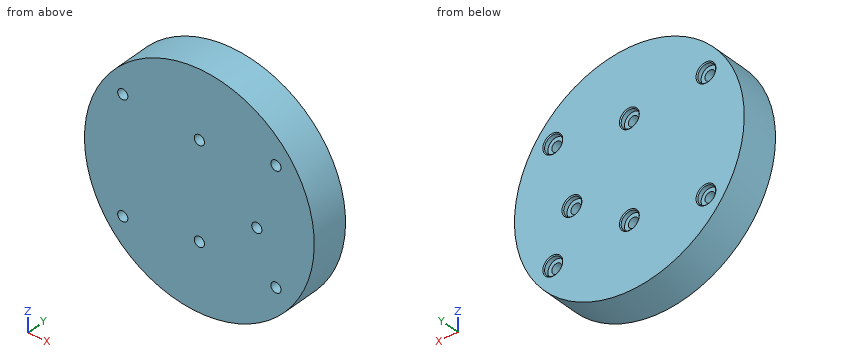
from build123d import *

# Parameters (mm, degrees)
SKETCH1_R                                     = 76.2
BOSS_EXTRUDE1_DEPTH                           = 25.4
CBORE_FOR_1_4_BUTTON_HEAD_CAP_SCREW1_AT_COUNT = 2
CBORE_FOR_1_4_BUTTON_HEAD_CAP_SCREW1_AT_PITCH = 45.790501198
CBORE_FOR_1_4_BUTTON_HEAD_CAP_SCREW1_2_COUNT  = 2
CBORE_FOR_1_4_BUTTON_HEAD_CAP_SCREW1_2_PITCH  = 63.5
CBORE_FOR_1_4_BUTTON_HEAD_CAP_SCREW1_3_COUNT  = 2
CBORE_FOR_1_4_BUTTON_HEAD_CAP_SCREW1_3_PITCH  = 86.36933773
CBORE_FOR_1_4_BUTTON_HEAD_CAP_SCREW1_4_COUNT  = 2
CBORE_FOR_1_4_BUTTON_HEAD_CAP_SCREW1_4_PITCH  = 51.195336702
CBORE_FOR_1_4_BUTTON_HEAD_CAP_SCREW1_5_COUNT  = 2
CBORE_FOR_1_4_BUTTON_HEAD_CAP_SCREW1_5_PITCH  = 51.195336702
CBORE_FOR_1_4_BUTTON_HEAD_CAP_SCREW1_6_COUNT  = 2
CBORE_FOR_1_4_BUTTON_HEAD_CAP_SCREW1_6_PITCH  = 86.36933773


with BuildPart() as part:
    # Sketch1 → Boss-Extrude1 (new body)
    with BuildSketch(Plane(origin=(0, 0, 0), x_dir=(1, 0, 0), z_dir=(0, 1, 0))):
        with Locations(Location((0, 0, 0), (0, 0, 270))):
            Circle(SKETCH1_R)
    extrude(amount=-BOSS_EXTRUDE1_DEPTH)

    # Sketch8 → CBORE for 1/4 Button Head Cap Screw1 (revolve, cut)
    with BuildSketch(Plane(origin=(0, 0, -31.75), x_dir=(0, 0, 1), z_dir=(1, 0, 0))):
        Polygon((0, 0), (0, 25.4), (3.3782, 25.4), (3.3782, 3.3528), (5.95376, 3.3528), (5.95376, 0.635), (6.58876, 0), align=None)
    cbore_for_1_4_button_head_cap_screw1 = revolve(axis=Axis((0, 6.35, -31.75), (0, -1, 0)), mode=Mode.SUBTRACT)

    # CBORE for 1/4 Button Head Cap Screw1 at: CBORE for 1/4 Button Head Cap Screw1 ×2
    with Locations(*[Vector(0.8320502943378437, 0, 0.5547001962252293) * (i * CBORE_FOR_1_4_BUTTON_HEAD_CAP_SCREW1_AT_PITCH) for i in range(1, CBORE_FOR_1_4_BUTTON_HEAD_CAP_SCREW1_AT_COUNT)]):
        add(cbore_for_1_4_button_head_cap_screw1, mode=Mode.SUBTRACT)

    # CBORE for 1_4 Button Head Cap Screw1 2: CBORE for 1/4 Button Head Cap Screw1 ×2
    with Locations(*[(0, 0, i * CBORE_FOR_1_4_BUTTON_HEAD_CAP_SCREW1_2_PITCH) for i in range(1, CBORE_FOR_1_4_BUTTON_HEAD_CAP_SCREW1_2_COUNT)]):
        add(cbore_for_1_4_button_head_cap_screw1, mode=Mode.SUBTRACT)

    # CBORE for 1_4 Button Head Cap Screw1 3: CBORE for 1/4 Button Head Cap Screw1 ×2
    with Locations(*[Vector(0.5881716976750462, 0, 0.8087360843031886) * (i * CBORE_FOR_1_4_BUTTON_HEAD_CAP_SCREW1_3_PITCH) for i in range(1, CBORE_FOR_1_4_BUTTON_HEAD_CAP_SCREW1_3_COUNT)]):
        add(cbore_for_1_4_button_head_cap_screw1, mode=Mode.SUBTRACT)

    # CBORE for 1_4 Button Head Cap Screw1 4: CBORE for 1/4 Button Head Cap Screw1 ×2
    with Locations(*[Vector(0.9922778767136676, 0, -0.12403473458920865) * (i * CBORE_FOR_1_4_BUTTON_HEAD_CAP_SCREW1_4_PITCH) for i in range(1, CBORE_FOR_1_4_BUTTON_HEAD_CAP_SCREW1_4_COUNT)]):
        add(cbore_for_1_4_button_head_cap_screw1, mode=Mode.SUBTRACT)

    # CBORE for 1_4 Button Head Cap Screw1 5: CBORE for 1/4 Button Head Cap Screw1 ×2
    with Locations(*[Vector(-0.9922778767136676, 0, -0.12403473458920862) * (i * CBORE_FOR_1_4_BUTTON_HEAD_CAP_SCREW1_5_PITCH) for i in range(1, CBORE_FOR_1_4_BUTTON_HEAD_CAP_SCREW1_5_COUNT)]):
        add(cbore_for_1_4_button_head_cap_screw1, mode=Mode.SUBTRACT)

    # CBORE for 1_4 Button Head Cap Screw1 6: CBORE for 1/4 Button Head Cap Screw1 ×2
    with Locations(*[Vector(-0.5881716976750463, 0, 0.8087360843031884) * (i * CBORE_FOR_1_4_BUTTON_HEAD_CAP_SCREW1_6_PITCH) for i in range(1, CBORE_FOR_1_4_BUTTON_HEAD_CAP_SCREW1_6_COUNT)]):
        add(cbore_for_1_4_button_head_cap_screw1, mode=Mode.SUBTRACT)


solid = part.part
The listing builds one solid part. Answer for the finished solid, in the listing's coordinates (mm). Coordinates: 2 decimals unless noted, no trailing zeros. Write each loop counter-clockwise with the first axis right and the second up, starting at its lowest first coordinate (ties: lowest second). Pieces come first, ordered by that corner, then holes. Notation, with made-up numbers: (-38, 6) -> (-2, 6) arc R37 cw to (-2, 45) -> close; hole circle Ø2 at (14.25, 84). An arc over 180 degrees is marked (long way). One line per question, with ' | ' between items.
1. Straight lines are drawn through the part: line 1 (Z direction, x = -53.5, y = -8); line 2 (Z direction, x = 52.5, y = -18); line 3 (X direction, y = -2.3, z = -6.35). For each, find the intervals that lie inside material, in ascending order.
Verdict:
line 1: z = -54.26 to -40.13, -36.07 to 36.07, 40.13 to 54.26 | line 2: z = -55.23 to -41.02, -35.18 to 35.18, 41.02 to 55.23 | line 3: x = -75.93 to 32.15, 44.05 to 75.93
2. Section A-A (x = 0) is taken. Determine the outline of the cut face in (y, z) (3 decimals), and give its area (3 significant figures).
Verdict:
outline: (-25.4, -76.2) -> (0, -76.2) -> (0, -38.339) -> (-0.635, -37.704) -> (-3.353, -37.704) -> (-3.353, -35.128) -> (-25.4, -35.128) -> close; (-25.4, -28.372) -> (-3.353, -28.372) -> (-3.353, -25.796) -> (-0.635, -25.796) -> (0, -25.161) -> (0, 25.161) -> (-0.635, 25.796) -> (-3.353, 25.796) -> (-3.353, 28.372) -> (-25.4, 28.372) -> close; (-25.4, 35.128) -> (-3.353, 35.128) -> (-3.353, 37.704) -> (-0.635, 37.704) -> (0, 38.339) -> (0, 76.2) -> (-25.4, 76.2) -> close | area: 3,490 mm^2
3. Section C-C (x = 38.1) is taken. Determine the outline of the cut face in (y, z) (3 decimals), and give its area (3 significant figures).
Verdict:
outline: (-25.4, -65.991) -> (0, -65.991) -> (0, -12.939) -> (-0.635, -12.304) -> (-3.353, -12.304) -> (-3.353, -9.728) -> (-25.4, -9.728) -> close; (-25.4, -2.972) -> (-3.353, -2.972) -> (-3.353, -0.396) -> (-0.635, -0.396) -> (0, 0.239) -> (0, 65.991) -> (-25.4, 65.991) -> close | area: 3,160 mm^2
4. Section D-D (z = -6.35) is taken. Determine the outline of the cut face in (x, y) (3 decimals), and give its area (3 significant figures).
Verdict:
outline: (-75.935, -25.4) -> (34.722, -25.4) -> (34.722, -3.353) -> (32.146, -3.353) -> (32.146, -0.635) -> (31.511, 0) -> (-75.935, 0) -> close; (41.478, -25.4) -> (75.935, -25.4) -> (75.935, 0) -> (44.689, 0) -> (44.054, -0.635) -> (44.054, -3.353) -> (41.478, -3.353) -> close | area: 3,670 mm^2
5. Section B-B (y = -20.75) is taken. Determine the outline of the cut face in (x, z).
Verdict:
outline: circle Ø152.4 at (0, 0); hole circle Ø6.76 at (-50.8, -38.1); hole circle Ø6.76 at (-50.8, 38.1); hole circle Ø6.76 at (0, -31.75); hole circle Ø6.76 at (0, 31.75); hole circle Ø6.76 at (38.1, -6.35); hole circle Ø6.76 at (50.8, -38.1); hole circle Ø6.76 at (50.8, 38.1)
6. Given pin 1 Ø19 at (x, z) = (50.8, -38.1) entering from +Y; pin 2 Ø3.5 at (x, z) = (-52, 38.5) entering from +Y; pin 3 Ø8 at (x, y) = (35.5, -7.5) entering from -Z; pin 4 Ø3.5 at (x, z) = (-49.5, -37) entering from +Y, each flat-ended and moving along its own axis, determine where each tip first touches the part or whether it passes through.
Verdict:
pin 1: stops at y = 0 | pin 2: passes through | pin 3: stops at z = -69.38 | pin 4: stops at y = -3.35
